Check sheet for the modelled part. Datum: model origin and axes. Units: mm. Round coordinates to 2 decimals unless told otherwise and drop trailing zeros. Order: outer loops, then holes, each group sorted by start corner. A loop starts at its lowest first (then second) coordinate and runs counter-clockwise, first axis right, second up. Notation, with made-up numbers: (-5.5, 57.5) -> (20.5, 57.5) arc R20 cw to (20.5, 95.5) -> close; hole circle Ø3 at (-15, 41). An arc over 180 degrees is marked (long way). Answer in a Markdown table with one row per item.
from build123d import *

# Parameters (mm, degrees)
SKETCH_1_W      = 10
SKETCH_1_H      = 10
EXTRUDE_1_DEPTH = 10


with BuildPart() as part:
    # Эскиз1 → Бобышка-Вытянуть1 (new body)
    with BuildSketch(Plane(origin=(0, 0, 0), x_dir=(1, 0, 0), z_dir=(0, 1, 0))):
        Polygon((-60, 0), (-15, 0), (-15, -900), (-5, -900), (-5, -890), (5, -890), (5, -900), (15, -900), (15, 0), (60, 0), (40, 45.461538462), (5, 45.461538462), (5, 25), (-5, 25), (-5, 45.461538462), (-40, 45.461538462), align=None)
        with Locations((0, -865)):
            Rectangle(SKETCH_1_W, SKETCH_1_H, mode=Mode.SUBTRACT)
        with Locations((0, -835)):
            Rectangle(SKETCH_1_W, SKETCH_1_H, mode=Mode.SUBTRACT)
        with Locations((0, -805)):
            Rectangle(SKETCH_1_W, SKETCH_1_H, mode=Mode.SUBTRACT)
        with Locations((0, -775)):
            Rectangle(SKETCH_1_W, SKETCH_1_H, mode=Mode.SUBTRACT)
        with Locations((0, -745)):
            Rectangle(SKETCH_1_W, SKETCH_1_H, mode=Mode.SUBTRACT)
        with Locations((0, -715)):
            Rectangle(SKETCH_1_W, SKETCH_1_H, mode=Mode.SUBTRACT)
        with Locations((0, -685)):
            Rectangle(SKETCH_1_W, SKETCH_1_H, mode=Mode.SUBTRACT)
        with Locations((0, -655)):
            Rectangle(SKETCH_1_W, SKETCH_1_H, mode=Mode.SUBTRACT)
        with Locations((0, -625)):
            Rectangle(SKETCH_1_W, SKETCH_1_H, mode=Mode.SUBTRACT)
        with Locations((0, -595)):
            Rectangle(SKETCH_1_W, SKETCH_1_H, mode=Mode.SUBTRACT)
        with Locations((0, -565)):
            Rectangle(SKETCH_1_W, SKETCH_1_H, mode=Mode.SUBTRACT)
        with Locations((0, -535)):
            Rectangle(SKETCH_1_W, SKETCH_1_H, mode=Mode.SUBTRACT)
        with Locations((0, -505)):
            Rectangle(SKETCH_1_W, SKETCH_1_H, mode=Mode.SUBTRACT)
    extrude(amount=EXTRUDE_1_DEPTH)


solid = part.part
Item 1: Scan lines: line 1 (X direction, y = 6.5, z = 566); line 2 (X direction, y = 4.75, z = 55.5); line 3 (Z direction, x = 18, y = 2.5). Record each from-to range of solid material in increasing order. Write a range as [from, to].
Result sheet:
| item | result |
|---|---|
| line 1 | x = [-15, -5], [5, 15] |
| line 2 | x = [-15, 15] |
| line 3 | z = [-45.46, 0] |
Item 2: Cross-section at A-A (y = 8). State how many separate pieces and enclosed holes the cut face has, and give its area (3 significant figures).
Result sheet:
| item | result |
|---|---|
| separate pieces | 1 |
| enclosed holes | 13 |
| area | 29,900 mm^2 |
Item 3: Cross-section at B-B (x = 27). Record the boundary of the cut face in (y, z), and give its area (3 significant figures).
Result sheet:
| item | result |
|---|---|
| outline | (0, -45.46) -> (10, -45.46) -> (10, 0) -> (0, 0) -> close |
| area | 455 mm^2 |
Item 4: Cross-section at C-C (z = 214). Record the boundary of the cut face in (x, y), and give its area (3 significant figures).
Result sheet:
| item | result |
|---|---|
| outline | (-15, 0) -> (15, 0) -> (15, 10) -> (-15, 10) -> close |
| area | 300 mm^2 |
Item 5: Depth check by flat-ended pin: P1, Ø1, axis at y = 2.5, z = 99, coming from the -X side; P2, Ø3, axis at x = -41.5, y = 7, coming from the +Z side; P3, Ø5, axis at y = 2.5, z = 575, coming from the +X side; P4, Ø10, axis at x = -22.5, z = 755, coming from the +Y side. Enter the tip coordinate at first touch or a pass-through.
Result sheet:
| item | result |
|---|---|
| P1 | stops at x = -15 |
| P2 | stops at z = 0 |
| P3 | stops at x = 15 |
| P4 | passes through |
